Autodesk Inventor part; units mm, degrees
ref_plane "YZ Plane" through (0, 0, 0) normal (1, 0, 0) x (0, 1, 0)
ref_plane "XZ Plane" through (0, 0, 0) normal (0, 1, 0) x (-1, 0, 0)
ref_plane "XY Plane" through (0, 0, 0) normal (0, 0, 1) x (1, 0, 0)
sketch "Sketch1" plane through (0, 0, 0) normal (0, 0, 1) x (1, 0, 0)
  line L0 (0, 0) -> (25.4, 0)
  line L1 (25.4, 0) -> (25.4, 25.4)
  line L2 (25.4, 25.4) -> (0, 25.4)
  line L3 (0, 25.4) -> (0, 0)
  line L4 (3.175, 3.175) -> (22.225, 3.175)
  line L5 (22.225, 3.175) -> (22.225, 22.225)
  line L6 (22.225, 22.225) -> (3.175, 22.225)
  line L7 (3.175, 22.225) -> (3.175, 3.175)
  dimension "d0" = 25.4
  dimension "d1" = 25.4
  dimension "d2" = 3.175
extrude "Extrusion1" add sketch "Sketch1" against normal blind 431.8
sketch "Sketch2" plane through (0, 0, 0) normal (-1, 0, 0) x (0, 0, 1)
  line L0 (-431.8, 25.4) -> (-431.8, 0)
  line L1 (0, 25.4) -> (0, 0)
  point P0 (-304.8, 12.7)
  point P1 (-279.4, 12.7)
  point P2 (-330.2, 12.7)
  point P3 (-101.6, 12.7)
  point P4 (-127, 12.7)
  point P5 (-152.4, 12.7)
  dimension "d5" = 25.4
  dimension "d6" = 25.4
  dimension "d7" = 101.6
  dimension "d25" = 101.6
  dimension "d26" = 25.4
  dimension "d27" = 25.4
hole "Hole1" at (0, 12.7, -304.8) at (0, 12.7, -279.4) at (0, 12.7, -330.2) at (0, 12.7, -127) at (0, 12.7, -101.6) at (0, 12.7, -152.4) direction (1, 0, 0) diameter 6.35 depth 25.4 tip angle 118
sketch "Sketch3" plane through (0, 0, 0) normal (0, -1, 0) x (1, 0, 0)
  line L0 (0, -431.8) -> (25.4, -431.8)
  line L1 (0, 0) -> (25.4, 0)
  point P0 (12.7, -330.2)
  point P1 (12.7, -355.6)
  point P2 (12.7, -381)
  point P3 (12.7, -50.8)
  point P4 (12.7, -76.2)
  point P5 (12.7, -101.6)
  point P6 (12.7, -419.1)
  point P7 (12.7, -12.7)
  dimension "d15" = 25.4
  dimension "d16" = 25.4
  dimension "d17" = 50.8
  dimension "d28" = 50.8
  dimension "d29" = 25.4
  dimension "d30" = 25.4
  dimension "d31" = 12.7
  dimension "d32" = 12.7
hole "Hole2" at (12.7, 0, -330.2) at (12.7, 0, -355.6) at (12.7, 0, -381) at (12.7, 0, -101.6) at (12.7, 0, -76.2) at (12.7, 0, -50.8) at (12.7, 0, -419.1) at (12.7, 0, -12.7) direction (0, 1, 0) diameter 6.35 depth 25.4 tip angle 118
properties part number "tower horizontal brace 17.5in"
Geometry: final body of the model. Coordinates: model frame, mm. A direction names the side the tool comes from. Give positions to 0.01 mm unless a question says otherwise; leave off trailing zeros. Loops run counter-clockwise (first coordinate to the right, second up) from the corner with the lowest first, then second, coordinate; pieces in that order, holes last. Notation, with made-up numbers: M 78.25,75.5 L 103.25,75.5 A32 ccw 103.25,111.5 Z; hole C 41.25,-2 d7. An arc over 180 degrees is marked long. Put each result on its own line as item: value.
1) Mould query, pull axis Y, two halves, no side actions, for faces 3 (the flat face through (13, 25.4, -213)), 4 (the flat face through (25.4, 13, -213)), 5 (the flat face through (22.225, 13, -213)). Classes: released by +Y, released by -Y, zero draft, split by the parting line, or undercut.
Computed values:
face 3: released by +Y
face 4: zero draft
face 5: undercut
2) Cut plane A-A, the plane z = -373. Return the cut outline in (x, y) (3 decimals).
Computed values:
outline: M 0,0 L 25.4,0 L 25.4,25.4 L 0,25.4 Z; hole M 3.175,3.175 L 22.225,3.175 L 22.225,22.225 L 3.175,22.225 Z
3) Material intervals for L1, parallel to X at y = 5.5, z = -281 (3 decimals); L2, parallel to X at y = 23.15, z = -355.6 (3 decimals), sorted ascending. Write a range as from..to.
Computed values:
L1: x = 0..3.175, 22.225..25.4
L2: x = 0..9.525, 15.875..25.4
4) First-contact query: P1, Ø5, axis at x = 13, y = 19, coming from the +Z side. Flat tip, straight axial feed; report the tip coordinate or a pass-through.
Computed values:
P1: passes through
5) Reachability of faces 1 (the flat face through (24, 13, -431.8)), 2 (the flat face through (13, 22.225, -213)) from +Z, -Z, +X, -X, +Y, -Y: full face, straight path, thin tool, end or side. Return the list, or none.
Computed values:
face 1: -Z, +X, -X, +Y, -Y
face 2: +Z, -Z
